Model file for the job. Use its own axes, mm. Face numbers are marked on the shaded views. A direction names the side the tool comes from. Coordinates: 2 decimals unless noted, no trailing zeros. Write each loop counter-clockwise with the first axis right and the second up, starting at its lowest first coordinate (ties: lowest second). Pieces come first, ordered by that corner, then holes. Notation, with made-up numbers: M 75,61 L 125,61 A33 ccw 125,95 Z; hole C -14,54 d1. An arc over 180 degrees is marked long. Answer in a Markdown table with one row per item. Add a question column.
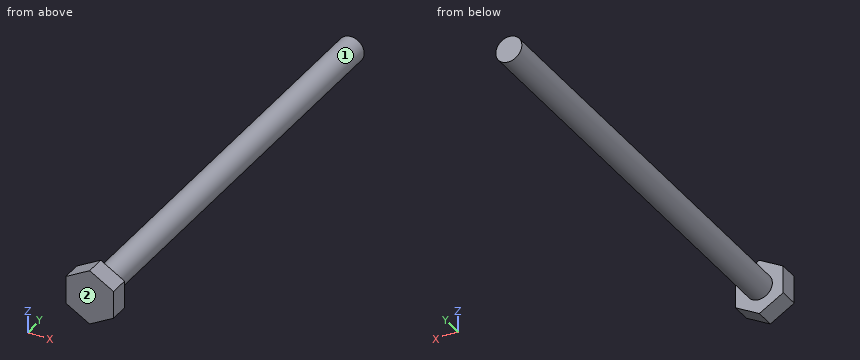
```python
from build123d import *

# Parameters (mm, degrees)
SKETCH_1_R      = 1.5
EXTRUDE_3_DEPTH = 50
EXTRUDE_START   = -2.2
SKETCH_1_4_R    = 1.5
EXTRUDE_4_DEPTH = 2.2


with BuildPart() as part:
    # Sketch 1 → Extrude 3 (new body)
    with BuildSketch(Plane(origin=(0, 0, 0), x_dir=(1, 0, 0), z_dir=(0, 1, 0))):
        with Locations(Location((0, 0, 0), (0, 0, 270))):
            Circle(SKETCH_1_R)
    extrude(amount=EXTRUDE_3_DEPTH)

    # Sketch 1_4 → Extrude 4 (add)
    # profile 1 of 2: a face of its own
    with BuildSketch(Plane(origin=(0, 0, 0), x_dir=(1, 0, 0), z_dir=(0, 1, 0)).offset(EXTRUDE_START)):
        Polygon((-2.75, 1.58771324), (-2.75, -1.58771324), (0, -3.175426481), (2.75, -1.58771324), (2.75, 1.58771324), (0, 3.175426481), align=None)
        with Locations(Location((0, 0, 0), (0, 0, 270))):
            Circle(SKETCH_1_4_R, mode=Mode.SUBTRACT)
    # profile 2 of 2: a face of its own
    with BuildSketch(Plane(origin=(0, 0, 0), x_dir=(1, 0, 0), z_dir=(0, 1, 0)).offset(EXTRUDE_START)):
        with Locations(Location((0, 0, 0), (0, 0, 270))):
            Circle(SKETCH_1_4_R)
    extrude(amount=EXTRUDE_4_DEPTH)


solid = part.part
```
1) Which spindle directions (+Z, -Z, +X, -X, +Y, -Y) get a long thin tool onto all of the face, cutting with end or side? Do the marked faces 1 and 2. Say none if no direction does.
2) Slice it at A-A (z = 0). Give the cut face in (x, y).
3) Drill centre lines: probe 1 along X at (y, z) = (38, 0); probe 2 along Y at (x, z) = (-1.4, -0.75); probe 3 along Z at (x, y) = (0.15, 21). Where is each one in solid material? Low to high.
4) Flat gauge pins, fed straight in: pin 1 Ø3 at (x, y) = (1.5, 29) entering from +Z; pin 2 Ø3 at (y, z) = (26.5, 0.5) entering from -X; pin 3 Ø3 at (x, y) = (0, 23.5) entering from -Z. Where does each tip first touch, or does it go through?
5) Slice it at B-B (x = 0.8). Give the cut face in (y, z).
6) Slice it at C-C (y = 41.5). Give the cut face in (x, z), then the cut area to 3 significant figures.
Ans:
| question | item | result |
|---|---|---|
| 1 | face 1 | +Y |
| 1 | face 2 | +Z, -Z, +X, -X, -Y |
| 2 | outline | M -2.75,-2.2 L 2.75,-2.2 L 2.75,0 L 1.5,0 L 1.5,50 L -1.5,50 L -1.5,0 L -2.75,0 Z |
| 3 | probe 1 | x = -1.5 to 1.5 |
| 3 | probe 2 | y = -2.2 to 0 |
| 3 | probe 3 | z = -1.49 to 1.49 |
| 4 | pin 1 | stops at z = 1.5 |
| 4 | pin 2 | stops at x = -1.5 |
| 4 | pin 3 | stops at z = -1.5 |
| 5 | outline | M -2.2,-2.71 L 0,-2.71 L 0,-1.27 L 50,-1.27 L 50,1.27 L 0,1.27 L 0,2.71 L -2.2,2.71 Z |
| 6 | outline | C 0,0 d3 |
| 6 | area | 7.07 mm2 |
